Input: part model. Units: mm. Frame: model coordinates. A direction names the side the tool comes from. Round coordinates to 2 decimals unless told otherwise and drop trailing zeros. Order: outer loops, then holes, each group sorted by start corner. A loop starts at its lowest first (then second) coordinate and runs counter-clockwise, first axis right, second up. Notation, with made-up numbers: (23, 13) -> (66, 13) arc R11 ccw to (66, 26) -> close; hole circle Ø6 at (-28, 29.25). An arc over 180 degrees is marked (long way). Answer as CSV lines item,"result". Start each with the question number.
1) Mould query, pull axis X, two halves, no side actions, for faces 3 (the face through (-1.5, -0.07, 9.51)), 4 (the face through (0.68, 1.15, 0.09)), 5 (the face through (2, 0, 0)), 6 (the face through (0.63, -1.08, 1.14)). Classes: +X half, -X half, draft (parallel to the pull), parting line (faces both ways), or undercut.
2) First-contact query: P1, Ø1.5, axis at y = 0.5, z = 8.5, coming from the -X side; P2, Ø1.5, axis at x = 1.5, z = 9.5, coming from the +Y side; P3, Ø3, axis at x = 0.5, z = 5, coming from the +Y side. Flat tips, straight axial feed; report the tip coordinate or a pass-through.
3) Access query for faces 1 (the face through (0, 0, 18)), 2 (the face through (0, 0, 2)). Directions: +Z, -Z, +X, -X, +Y, -Y. A direction counts if a zero-diameter tool reaches every point of the face in a straight line with its end or side. Return the directions, or none.
4) Section query B-B, the plane z = 10.25. Output: boundary loops of the cut face in (x, y).
5) Section query A-A, the plane y = 0. Output: boundary loops of the cut face in (x, z), and give its area (3 significant figures).
6) Line query: L1, parallel to X at y = 0.4, z = 5.25; L2, parallel to Y at x = -0.05, z = 6; L3, parallel to X at y = -0.9, z = 9. Output: solid intervals per line, ascending.
```python
from build123d import *

# Parameters (mm, degrees)
SKETCH1_R           = 2.75
BOSS_EXTRUDE1_DEPTH = 2
SKETCH2_R           = 1.5
BOSS_EXTRUDE2_DEPTH = 16
CHAMFER1_SIZE       = 1.5
FILLET1_R           = 0.3
CHAMFER2_SIZE       = 0.5
CUT_EXTRUDE1_DEPTH  = 2
FILLET2_R           = 0.3


with BuildPart() as part:
    # Sketch1 → Boss-Extrude1 (new body)
    with BuildSketch(Plane.XY):
        Circle(SKETCH1_R)
    extrude(amount=BOSS_EXTRUDE1_DEPTH)

    # Sketch2 → Boss-Extrude2 (add)
    with BuildSketch(Plane.XY.offset(2)):
        Circle(SKETCH2_R)
    extrude(amount=BOSS_EXTRUDE2_DEPTH)

    # Chamfer1
    # the kernel refuses this chamfer: 1.5 mm, written as the material it takes off along each edge
    with BuildSketch(Plane(origin=(0, 0, 2), x_dir=(1, 0, 0), z_dir=(0, -1, 0))) as chamfer1_piece_1_section:
        Polygon((2.75, -CHAMFER1_SIZE), (2.75 - CHAMFER1_SIZE, 0), (2.75, 0), align=None)
    chamfer1_piece_1 = revolve(axis=Axis((0, 0, 2), (0, 0, 1)), mode=Mode.PRIVATE)
    chamfer1_piece_1 = chamfer1_piece_1 - Plane(origin=(0, 0, 1.122011251), x_dir=(1, 0, 0), z_dir=(0, 0, -1)) * Cylinder(1.5, 11, mode=Mode.PRIVATE)
    add(chamfer1_piece_1, mode=Mode.SUBTRACT)

    # Fillet1
    fillet1_edges = [part.edges().sort_by_distance(p)[0] for p in [
        (-2.75, 0, 0),
    ]]
    fillet(fillet1_edges, radius=FILLET1_R)

    # Chamfer2
    chamfer2_edges = [part.edges().sort_by_distance(p)[0] for p in [
        (-1.5, 0, 18),
    ]]
    chamfer(chamfer2_edges, length=CHAMFER2_SIZE)

    # Sketch3 → Cut-Extrude1 (cut)
    with BuildSketch(Plane(origin=(0, 0, 0), x_dir=(-1, 0, 0), z_dir=(0, 0, -1))):
        Polygon((0, -1.443375673), (1.25, -0.721687836), (1.25, 0.721687836), (0, 1.443375673), (-1.25, 0.721687836), (-1.25, -0.721687836), align=None)
    extrude(amount=-CUT_EXTRUDE1_DEPTH, mode=Mode.SUBTRACT)

    # Fillet2
    fillet2_edges = [part.edges().sort_by_distance(p)[0] for p in [
        (0.625, -1.082531755, 0),
        (-0.625, -1.082531755, 0),
        (-1.25, 0, 0),
        (-0.625, 1.082531755, 0),
        (0.625, 1.082531755, 0),
        (1.25, 0, 0),
    ]]
    fillet(fillet2_edges, radius=FILLET2_R)


solid = part.part
```
Findings:
1,face 3,"parting line"
1,face 4,"undercut"
1,face 5,"draft"
1,face 6,"undercut"
2,P1,"stops at x = -1.5"
2,P2,"stops at y = 1.3"
2,P3,"stops at y = 1.5"
3,face 1,"+Z, +X, -X, +Y, -Y"
3,face 2,"-Z"
4,outline,"circle Ø3 at (0, 0)"
5,outline,"(-2.75, 0.3) arc R0.3 ccw to (-2.45, 0) -> (-1.55, 0) arc R0.3 ccw to (-1.25, 0.3) -> (-1.25, 2) -> (1.25, 2) -> (1.25, 0.3) arc R0.3 ccw to (1.55, 0) -> (2.45, 0) arc R0.3 ccw to (2.75, 0.3) -> (2.75, 0.5) -> (1.5, 1.75) -> (1.5, 17.5) -> (1, 18) -> (-1, 18) -> (-1.5, 17.5) -> (-1.5, 1.75) -> (-2.75, 0.5) -> close"
5,area,"51.5 mm^2"
6,L1,"x = -1.45 to 1.45"
6,L2,"y = -1.5 to 1.5"
6,L3,"x = -1.2 to 1.2"
